Read the model definition and answer for the solid it produces. Units are mm, in the model's axes. A direction names the side the tool comes from. Coordinates: 2 decimals unless noted, no trailing zeros. Loops run counter-clockwise (first coordinate to the right, second up) from the corner with the lowest first, then second, coordinate; pieces in that order, holes last. Notation, with made-up numbers: (-23.75, -2.75) -> (-3.75, -2.75) arc R20 ccw to (-3.75, 8.25) -> close; hole circle Ø8 at (78.5, 58.25). An arc over 180 degrees is marked (long way). Answer as a JSON object with one key per item and string values. Group by question number.
Q1. The part is cut by section D-D on y = 0.65. State how many separate pieces and enclosed holes the cut face has, and give its area (3 significant figures).
Q2. For faces 1 (the flat face through (-94, 1.588, -133)), 2 (the flat face through (-60, 1, -155)), determine the directions among +Z, -Z, +X, -X, +Y, -Y from which every point of the face is accessible in a straight line to the end or side of a thin tool.
Q3. Determine the mould class of faces 3 (the flat face through (-96, 0, -133)), 4 (the flat face through (-90, 1, -155)) for opening direction X: released by +X, released by -X, zero draft, split by the parting line, or undercut.
Q4. The part is cut by section C-C on z = -90. Write down the section's boundary in (x, y).
Q5. The part is cut by section B-B on x = -145. Write down the section's boundary in (y, z).
Q6. Straight lines are drawn through the part: line 1 along Z through (x, y) = (-37, 0.8); line 2 along X through (y, z) = (0.9, -227); line 3 along Z through (x, y) = (-121.5, 1.35). For each, find the intervals that lie inside material, in ascending order. Write a range as [from, to].
Q7. The part is cut by section A-A on z = -255. Write down the section's boundary in (x, y), and give its area (3 significant figures).
Autodesk Inventor part; units mm, degrees
ref_plane "YZ Plane" through (0, 0, 0) normal (1, 0, 0) x (0, 1, 0)
ref_plane "XZ Plane" through (0, 0, 0) normal (0, 1, 0) x (-1, 0, 0)
ref_plane "XY Plane" through (0, 0, 0) normal (0, 0, 1) x (1, 0, 0)
sketch "Sketch1" plane through (0, 0, 0) normal (0, 1, 0) x (-1, 0, 0)
  line L0 (0, 0) -> (190, 0)
  line L1 (190, 0) -> (190, -270)
  line L2 (190, -270) -> (0, -270)
  line L3 (0, -270) -> (0, 0)
  line L4 (180, -10) -> (160, -10)
  line L5 (160, -10) -> (160, -30)
  line L6 (160, -30) -> (180, -30)
  line L7 (180, -30) -> (180, -10)
  line L8 (150, -10) -> (130, -10)
  line L9 (130, -10) -> (130, -30)
  line L10 (130, -30) -> (150, -30)
  line L11 (150, -30) -> (150, -10)
  line L12 (120, -10) -> (100, -10)
  line L13 (100, -10) -> (100, -30)
  line L14 (100, -30) -> (120, -30)
  line L15 (120, -30) -> (120, -10)
  line L16 (90, -10) -> (70, -10)
  line L17 (70, -10) -> (70, -30)
  line L18 (70, -30) -> (90, -30)
  line L19 (90, -30) -> (90, -10)
  line L20 (60, -10) -> (40, -10)
  line L21 (40, -10) -> (40, -30)
  line L22 (40, -30) -> (60, -30)
  line L23 (60, -30) -> (60, -10)
  line L24 (28.2524, -10) -> (8.2524, -10)
  line L25 (8.2524, -10) -> (8.2524, -30)
  line L26 (8.2524, -30) -> (28.2524, -30)
  line L27 (28.2524, -30) -> (28.2524, -10)
  circle A0 centre (165, -60) radius 6
  circle A1 centre (165, -90) radius 6
  circle A2 centre (165, -120) radius 6
  circle A3 centre (165, -150) radius 6
  circle A4 centre (165, -180) radius 6
  circle A5 centre (165, -210) radius 6
  line L28 (180, -260) -> (160, -260)
  line L29 (160, -260) -> (160, -240)
  line L30 (160, -240) -> (180, -240)
  line L31 (180, -240) -> (180, -260)
  line L32 (150, -260) -> (130, -260)
  line L33 (130, -260) -> (130, -240)
  line L34 (130, -240) -> (150, -240)
  line L35 (150, -240) -> (150, -260)
  line L36 (130, -50) -> (110, -50)
  line L37 (110, -50) -> (110, -70)
  line L38 (110, -70) -> (130, -70)
  line L39 (130, -70) -> (130, -50)
  line L40 (100, -80) -> (80, -80)
  line L41 (80, -80) -> (80, -100)
  line L42 (80, -100) -> (100, -100)
  line L43 (100, -100) -> (100, -80)
  line L44 (70, -70) -> (50, -70)
  line L45 (50, -70) -> (50, -50)
  line L46 (50, -50) -> (70, -50)
  line L47 (70, -50) -> (70, -70)
  line L48 (70, -110) -> (50, -110)
  line L49 (50, -110) -> (50, -130)
  line L50 (50, -130) -> (70, -130)
  line L51 (70, -130) -> (70, -110)
  line L52 (40, -80) -> (20, -80)
  line L53 (20, -80) -> (20, -100)
  line L54 (20, -100) -> (40, -100)
  line L55 (40, -100) -> (40, -80)
  line L56 (110, -110) -> (130, -110)
  line L57 (130, -110) -> (130, -130)
  line L58 (130, -130) -> (110, -130)
  line L59 (110, -130) -> (110, -110)
  line L60 (20, -260) -> (40, -260)
  line L61 (40, -260) -> (40, -240)
  line L62 (40, -240) -> (20, -240)
  line L63 (20, -240) -> (20, -260)
  line L64 (40, -230) -> (20, -230)
  line L65 (20, -230) -> (20, -210)
  line L66 (20, -210) -> (40, -210)
  line L67 (40, -210) -> (40, -230)
  line L68 (20, -200) -> (40, -200)
  line L69 (40, -200) -> (40, -180)
  line L70 (40, -180) -> (20, -180)
  line L71 (20, -180) -> (20, -200)
  line L72 (20, -170) -> (40, -170)
  line L73 (40, -170) -> (40, -150)
  line L74 (40, -150) -> (20, -150)
  line L75 (20, -150) -> (20, -170)
  line L76 (60, -260) -> (110, -260)
  line L77 (110, -260) -> (110, -210)
  line L78 (110, -210) -> (60, -210)
  line L79 (60, -210) -> (60, -260)
  line L80 (60, -200) -> (140, -200)
  line L81 (140, -200) -> (140, -186)
  line L82 (140, -186) -> (60, -186)
  line L83 (60, -186) -> (60, -200)
  line L84 (70, -170) -> (70, -150)
  line L85 (80, -150) -> (80, -170)
  line L86 (110, -170) -> (130, -170)
  line L87 (130, -170) -> (130, -150)
  line L88 (130, -150) -> (110, -150)
  line L89 (110, -150) -> (110, -170)
  line L90 (70, -150) -> (50, -160)
  line L91 (70, -170) -> (50, -160)
  line L92 (80, -150) -> (100, -160)
  line L93 (80, -170) -> (100, -160)
extrude "Extrusion1" add sketch "Sketch1" along normal blind 1.5875
sketch "Sketch2" plane through (-190, 0, 0) normal (0, 0, 1) x (1, 0, 0)
  line L0 (190, 0) -> (190, 1.5875)
  line L1 (0, 0) -> (0, 1.5875)
  line L2 (190, 1.5875) -> (0, 1.5875)
  line L3 (0, 1.5875) -> (0, 0)
  line L4 (0, 0) -> (190, 0)
  line L5 (190, 0) -> (190, 1.5875)
extrude "Extrusion2" add sketch "Sketch2" along normal blind 12.7
sketch "Sketch3" plane through (0, 0, -270) normal (0, 0, -1) x (-1, 0, 0)
  line L0 (190, 0) -> (0, 0)
  line L1 (0, 1.5875) -> (190, 1.5875)
  line L2 (0, 0) -> (190, 0)
  line L3 (190, 0) -> (190, 1.5875)
  line L4 (190, 1.5875) -> (0, 1.5875)
  line L5 (0, 1.5875) -> (0, 0)
  point P0 (0, 1.5875)
extrude "Extrusion3" add sketch "Sketch3" along normal blind 12.7
properties part number "Front Plywood"
Final values:
{
 "1": {"separate pieces": "1", "enclosed holes": "29", "area": "43,800 mm2"},
 "2": {"face 1": "+Z, -Z, +X, -X, +Y", "face 2": "+Y, -Y"},
 "3": {"face 3": "zero draft", "face 4": "undercut"},
 "4": {"outline": "(-190, 0) -> (-171, 0) -> (-171, 1.59) -> (-190, 1.59) -> close; (-159, 0) -> (-100, 0) -> (-100, 1.59) -> (-159, 1.59) -> close; (-80, 0) -> (-40, 0) -> (-40, 1.59) -> (-80, 1.59) -> close; (-20, 0) -> (0, 0) -> (0, 1.59) -> (-20, 1.59) -> close"},
 "5": {"outline": "(0, -282.7) -> (1.59, -282.7) -> (1.59, -260) -> (0, -260) -> close; (0, -240) -> (1.59, -240) -> (1.59, -30) -> (0, -30) -> close; (0, -10) -> (1.59, -10) -> (1.59, 12.7) -> (0, 12.7) -> close"},
 "6": {"line 1": "z = [-282.7, -260], [-240, -230], [-210, -200], [-180, -170], [-150, -100], [-80, 12.7]", "line 2": "x = [-190, -110], [-60, -40], [-20, 0]", "line 3": "z = [-282.7, -200], [-186, -170], [-150, -130], [-110, -70], [-50, 12.7]"},
 "7": {"outline": "(-190, 0) -> (-180, 0) -> (-180, 1.59) -> (-190, 1.59) -> close; (-160, 0) -> (-150, 0) -> (-150, 1.59) -> (-160, 1.59) -> close; (-130, 0) -> (-110, 0) -> (-110, 1.59) -> (-130, 1.59) -> close; (-60, 0) -> (-40, 0) -> (-40, 1.59) -> (-60, 1.59) -> close; (-20, 0) -> (0, 0) -> (0, 1.59) -> (-20, 1.59) -> close", "area": "127 mm2"}
}
